Source: three-view drawing plus pictorial views. Frame: mm from the lowest corner of the part. Give positions to 0.01 mm unless a question says otherwise; leave off trailing zeros. Order: outer loops, then holes, each group sorted by start corner. A loop starts at its lowest first (then second) coordinate and runs counter-clockwise, first axis right, second up.
1) Section A-A, the plane z = 1.6. Return loops of the section in (x, y), plus the area to 3 significant figures.
2) Material intervals for line 1 (X direction, y = 15, z = 1.3); line 2 (Y direction, x = 13, z = 0.1); line 3 (Y direction, x = 21, z = 1.45), sorted ascending.
3) First-contact query: P1, Ø2.5, axis at x = 165, y = 15, coming from the -Z side. Flat tip, straight axial feed; report the tip coordinate or a pass-through.
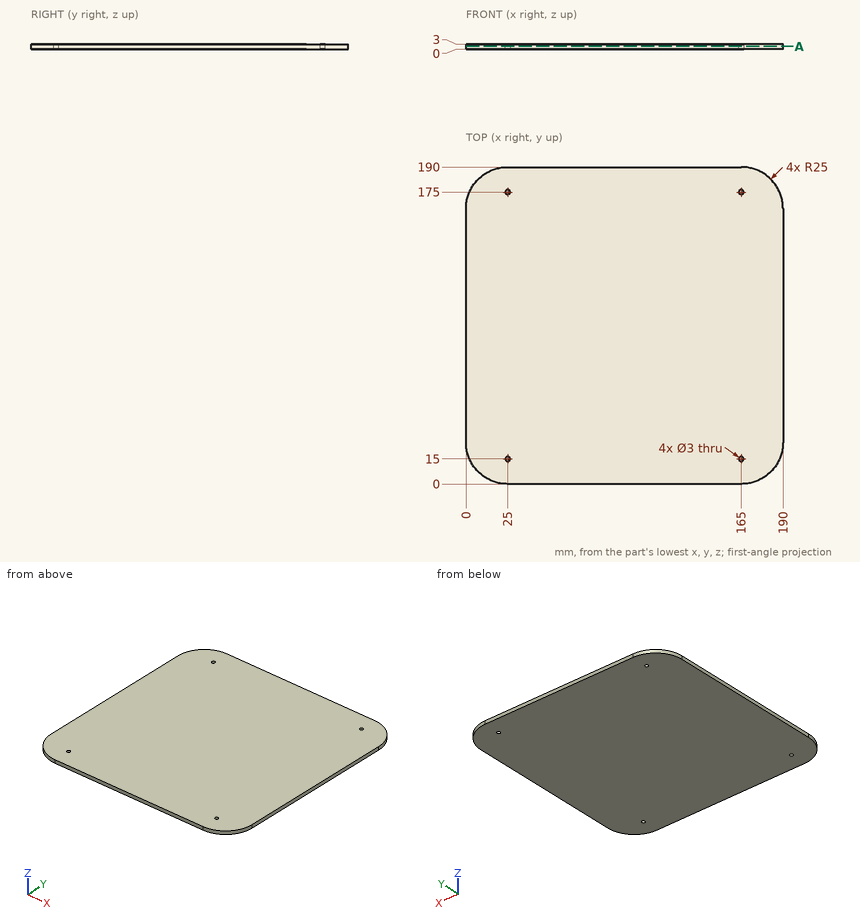
From the geometry:
1. outline: (0, 25) arc R25 ccw to (25, 0) - (165, 0) arc R25 ccw to (190, 25) - (190, 165) arc R25 ccw to (165, 190) - (25, 190) arc R25 ccw to (0, 165) - close; hole circle Ø3 at (25, 15); hole circle Ø3 at (25, 175); hole circle Ø3 at (165, 15); hole circle Ø3 at (165, 175)
1. area: 35,500 mm2
2. line 1: x = 2.09 to 23.5, 26.5 to 163.5, 166.5 to 187.91
2. line 2: y = 3.07 to 186.93
2. line 3: y = 0.32 to 189.68
3. P1: passes through
